from build123d import *

# Parameters (mm, degrees)
SKETCH1_W = 7
SKETCH1_H = 1
FILLET1_R = 1


with BuildPart() as part:
    # Sketch1 → Revolve1 (revolve)
    with BuildSketch(Plane.XY, mode=Mode.PRIVATE) as revolve1_sk:
        Polygon((-3.5, 2.5), (-3.5, 3.5), (-3.5, 6.25), (-5.5, 6.25), (-5.5, 2.5), align=None)
        with Locations((0, 3)):
            Rectangle(SKETCH1_W, SKETCH1_H)
    revolve(revolve1_sk.sketch.rotate(Axis((0, 0, 0), (1, 0, 0)), 90), axis=Axis((0, 0, 0), (1, 0, 0)))

    # Fillet1
    fillet1_edges = [part.edges().sort_by_distance(p)[0] for p in [
        (-3.5, 0, -3.5),
    ]]
    fillet(fillet1_edges, radius=FILLET1_R)


solid = part.part
Source: CAD feature listing. Evaluate the final solid. Frame: model axes, mm. Give positions to 0.01 mm unless a question says otherwise; leave off trailing zeros. Order: outer loops, then holes, each group sorted by start corner. A loop starts at its lowest first (then second) coordinate and runs counter-clockwise, first axis right, second up. Notation, with made-up numbers: (57.25, 48) -> (93.25, 48) arc R33 cw to (93.25, 85) -> close; hole circle Ø11 at (45, 52). An arc over 180 degrees is marked (long way). Write item = value, one per line.
Q1. Pull-direction query (Z, two-part tool) for faces 1 (the face through (0.542, 3.105, 1.615)), 2 (the face through (-3.5, 4, -3)), 3 (the face through (-0.9, -0.1, -2.5)); classes: released by +Z, released by -Z, zero draft, split by the parting line, or undercut.
Data:
face_1 = split by the parting line
face_2 = zero draft
face_3 = undercut
Q2. Cut plane D-D, the plane y = -5. Output: boundary loops of the cut face in (x, z), and give its area (3 significant figures).
Data:
outline = (-5.5, -3.75) -> (-3.5, -3.75) -> (-3.5, 3.75) -> (-5.5, 3.75) -> close
area = 15.0 mm^2
Q3. Cut plane C-C, the plane x = -3.75. Output: boundary loops of the cut face in (y, z), and give its area (3 significant figures).
Data:
outline = circle Ø12.5 at (0, 0); hole circle Ø5 at (0, 0)
area = 103 mm^2
Q4. Material intervals for line 1 (Y direction, x = -1, z = 0); line 2 (X direction, y = 1, z = 5.75); line 3 (Z direction, x = -2.5, y = 0.5), sorted ascending. Write a range as from..to.
Data:
line_1 = -3.5..-2.5, 2.5..3.5
line_2 = -5.5..-3.5
line_3 = -3.46..-2.45, 2.45..3.46
Q5. Pin query (flat end, axial travel): pin 1 (5 mm diameter, centred on x = -2.5, z = -2.5, fed in from -Y); pin 2 (1 mm diameter, centred on x = -1.5, z = 2, fed in from +Y). Return the tip coordinate at first contact, or that it passes through.
Data:
pin_1 = -6.25
pin_2 = 3.16
Q6. Cut plane A-A, the plane z = 0. Output: boundary loops of the cut face in (x, y), and give its area (3 significant figures).
Data:
outline = (-5.5, -6.25) -> (-3.5, -6.25) -> (-3.5, -4.5) arc R1 cw to (-2.5, -3.5) -> (3.5, -3.5) -> (3.5, -2.5) -> (-5.5, -2.5) -> close; (-5.5, 2.5) -> (3.5, 2.5) -> (3.5, 3.5) -> (-2.5, 3.5) arc R1 cw to (-3.5, 4.5) -> (-3.5, 6.25) -> (-5.5, 6.25) -> close
area = 29.4 mm^2
